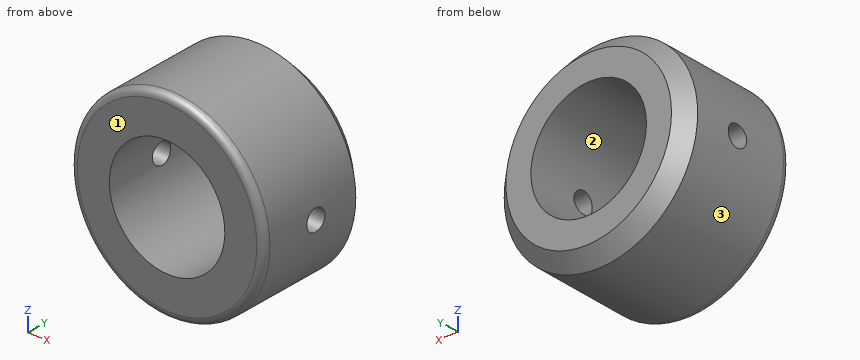
```python
from build123d import *

# Parameters (mm, degrees)
SKETCH1_W               = 2.8
SKETCH1_H               = 8.5
CHAMFER1_SIZE           = 1
CUT_EXTRUDE1_DEPTH      = 11.70829118
CUT_EXTRUDE1_DEPTH_BACK = 11.70829118
SKETCH3_R               = 0.75
FILLET1_R               = 0.5


with BuildPart() as part:
    # Sketch1 → Revolve1 (revolve)
    with BuildSketch(Plane(origin=(0, 0, 0), x_dir=(0, 0, -1), z_dir=(1, 0, 0)), mode=Mode.PRIVATE) as revolve1_sk:
        with Locations((5.55, 0)):
            Rectangle(SKETCH1_W, SKETCH1_H)
    revolve(revolve1_sk.sketch.rotate(Axis((0, 19.013157895, 0), (0, -1, 0)), 180), axis=Axis((0, 19.013157895, 0), (0, -1, 0)))

    # Chamfer1
    chamfer1_edges = [part.edges().sort_by_distance(p)[0] for p in [
        (0, 4.25, -6.95),
    ]]
    chamfer(chamfer1_edges, length=CHAMFER1_SIZE)

    # Sketch3 → Cut-Extrude1 (cut, two sides: drawn at the far end of the back side and taken through both)
    with BuildSketch(Plane(origin=(0, 0, 0), x_dir=(0, 0, -1), z_dir=(1, 0, 0)).offset(-CUT_EXTRUDE1_DEPTH_BACK)):
        Circle(SKETCH3_R)
    extrude(amount=CUT_EXTRUDE1_DEPTH + CUT_EXTRUDE1_DEPTH_BACK, mode=Mode.SUBTRACT)

    # Fillet1
    fillet1_edges = [part.edges().sort_by_distance(p)[0] for p in [
        (0, -4.25, -6.95),
    ]]
    fillet(fillet1_edges, radius=FILLET1_R)


solid = part.part
```
The model under review builds one solid part; all positions refer to its coordinate system, in mm. Face numbers are marked on the shaded views. Round coordinates to 2 decimals unless told otherwise and drop trailing zeros. Loops run counter-clockwise (first coordinate to the right, second up) from the corner with the lowest first, then second, coordinate; pieces in that order, holes last. Notation, with made-up numbers: (73, -37) -> (123, -37) arc R23 cw to (123, -24) -> close; hole circle Ø3 at (54.5, 6.5). An arc over 180 degrees is marked (long way). Answer in a Markdown table with one row per item.
1) For pin 1 Ø4 at (y, z) = (2, -4.5) entering from -X; pin 2 Ø1.2 at (y, z) = (0, 0) entering from +X; pin 3 Ø5 at (x, y) = (-4, 0) entering from -Z; pin 4 Ø1 at (x, y) = (4.5, 2) entering from +Z, all flat-tipped, find the tip position at first contact; note any pin that passes through.
Taken from the geometry:
| item | result |
|---|---|
| pin 1 | stops at x = -6.48 |
| pin 2 | passes through |
| pin 3 | stops at z = -6.79 |
| pin 4 | stops at z = 5.68 |
2) Consider section D-D, the plane y = 3.5. Write out the cut boundary in (x, z).
Taken from the geometry:
| item | result |
|---|---|
| outline | circle Ø13.4 at (0, 0); hole circle Ø8.3 at (0, 0) |
3) Draft analysis for pull direction Z (two halves, no side actions). For the marked faces 1, 2 and 3, state which applies: pulls with the +Z half, pulls with the -Z half, needs draft (parallel to the pull), parting line crosses it, or undercut.
Taken from the geometry:
| item | result |
|---|---|
| face 1 | needs draft |
| face 2 | undercut |
| face 3 | parting line crosses it |
4) Consider section C-C, the plane y = 0. Write out the cut boundary in (x, z).
Taken from the geometry:
| item | result |
|---|---|
| outline | (-6.91, -0.75) arc R6.95 ccw to (6.91, -0.75) -> (4.08, -0.75) arc R4.15 cw to (-4.08, -0.75) -> close; (-6.91, 0.75) -> (-4.08, 0.75) arc R4.15 cw to (4.08, 0.75) -> (6.91, 0.75) arc R6.95 ccw to start |
5) Consider section B-B, the plane z = 0. Write out the cut boundary in (x, y).
Taken from the geometry:
| item | result |
|---|---|
| outline | (-6.95, -3.75) arc R0.5 ccw to (-6.45, -4.25) -> (-4.15, -4.25) -> (-4.15, -0.75) -> (-6.95, -0.75) -> close; (-6.95, 0.75) -> (-4.15, 0.75) -> (-4.15, 4.25) -> (-5.95, 4.25) -> (-6.95, 3.25) -> close; (4.15, -4.25) -> (6.45, -4.25) arc R0.5 ccw to (6.95, -3.75) -> (6.95, -0.75) -> (4.15, -0.75) -> close; (4.15, 0.75) -> (6.95, 0.75) -> (6.95, 3.25) -> (5.95, 4.25) -> (4.15, 4.25) -> close |
6) Wall thickness on line 1 along Z through (x, y) = (3, -3); line 2 along Y through (x, z) = (-6, -0.5); line 3 along X through (y, z) = (2.25, -2): over which ranges is each line inside the solid? List them lowest first.
Taken from the geometry:
| item | result |
|---|---|
| line 1 | z = -6.27 to -2.87, 2.87 to 6.27 |
| line 2 | y = -4.25 to -0.56, 0.56 to 4.18 |
| line 3 | x = -6.66 to -3.64, 3.64 to 6.66 |
7) Consider section A-A, the plane x = 0. Write out the cut boundary in (y, z), plus the area to 3 significant figures.
Taken from the geometry:
| item | result |
|---|---|
| outline | (-4.25, -6.45) arc R0.5 ccw to (-3.75, -6.95) -> (3.25, -6.95) -> (4.25, -5.95) -> (4.25, -4.15) -> (-4.25, -4.15) -> close; (-4.25, 4.15) -> (4.25, 4.15) -> (4.25, 5.95) -> (3.25, 6.95) -> (-3.75, 6.95) arc R0.5 ccw to (-4.25, 6.45) -> close |
| area | 46.5 mm² |
